Here's the drawing with two shaded views (mm, measured from the low corner). I have some questions. Coordinates: 2 decimals unless noted, no trailing zeros. Loops run counter-clockwise (first coordinate to the right, second up) from the corner with the lowest first, then second, coordinate; pieces in that order, holes last.
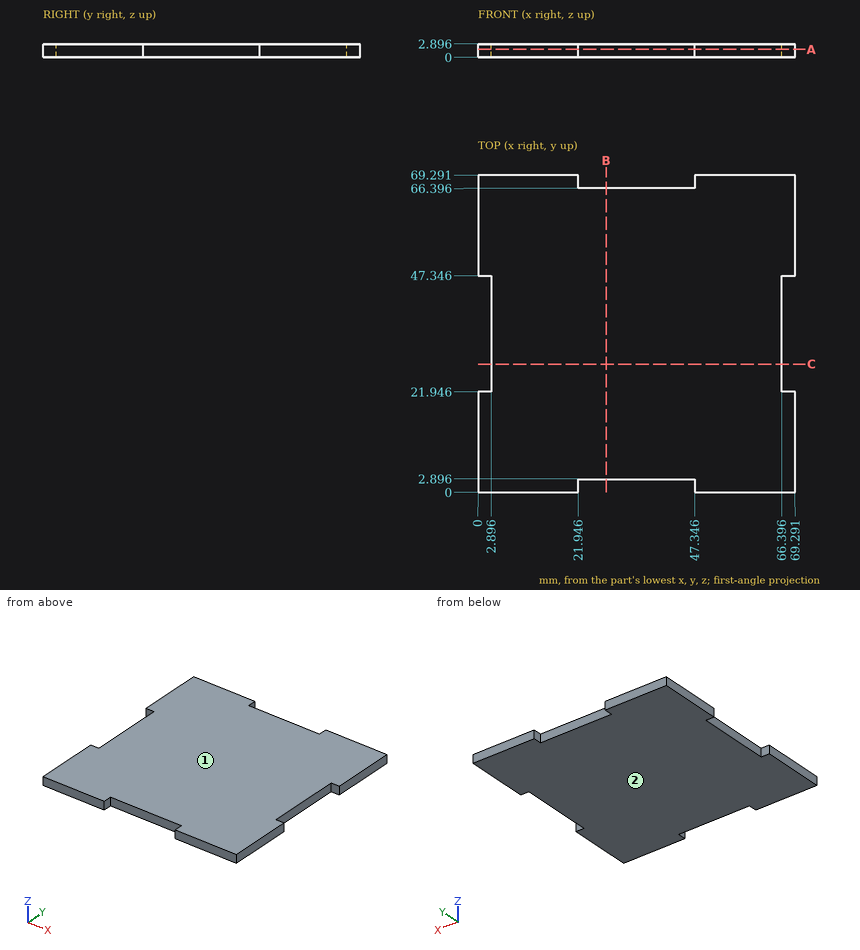
(1) If we mould it in two halves opening along Z, with no side actions, what happens to the marked faces 1 and 2? For each: released by +Z, released by -Z, zero draft, split by the parting line, or undercut.
Check values:
face 1: released by +Z
face 2: released by -Z
(2) I want a section at B-B on x = 28. Write out the boundary of the cut face in (y, z) (1 decimal), then the cut area to 3 significant figures.
Check values:
outline: (2.9, 0) - (66.4, 0) - (66.4, 2.9) - (2.9, 2.9) - close
area: 184 mm2
(3) If I drill on probe 1 along X at (y, z) = (66.5, 2.7) (1 decimal); probe 2 along X at (y, z) = (37, 2.45) (1 decimal), over which ranges is the centre line in solid material (lowest first)?
Check values:
probe 1: x = 0 to 21.9, 47.3 to 69.3
probe 2: x = 2.9 to 66.4
(4) I'm going to push flat-ended pins straight in: pin 1 (1.4 mm diameter, centred on y = 37.5, z = 2, fed in from -X); pin 2 (12 mm diameter, centred on x = 55, y = 11, fed in from -Z); pin 3 (0.9 mm diameter, centred on y = 34, z = 1, fed in from +X); pin 4 (1.4 mm diameter, centred on x = 31, z = 1.5, fed in from -Y). Where does each tip first touch, or does it pass through?
Check values:
pin 1: stops at x = 2.9
pin 2: stops at z = 0
pin 3: stops at x = 66.4
pin 4: stops at y = 2.9
(5) I want a section at A-A on z = 1.7. Write out the boundary of the cut face in (x, y) (1 decimal), then the cut area to 3 significant figures.
Check values:
outline: (0, 0) - (21.9, 0) - (21.9, 2.9) - (47.3, 2.9) - (47.3, 0) - (69.3, 0) - (69.3, 21.9) - (66.4, 21.9) - (66.4, 47.3) - (69.3, 47.3) - (69.3, 69.3) - (47.3, 69.3) - (47.3, 66.4) - (21.9, 66.4) - (21.9, 69.3) - (0, 69.3) - (0, 47.3) - (2.9, 47.3) - (2.9, 21.9) - (0, 21.9) - close
area: 4,510 mm2
